```python
from build123d import *

# Parameters (mm, degrees)
SKETCH2_R                       = 10
BOSS_EXTRUDE1_DEPTH             = 12.7
TAP_DRILL_FOR_M3X0_5_TAP1_D     = 2.5
TAP_DRILL_FOR_M3X0_5_TAP1_DEPTH = 25
TAP_DRILL_FOR_M3X0_5_TAP1_TIP   = 0.751075774
M4X0_7_TAPPED_HOLE1_D           = 3.3
M4X0_7_TAPPED_HOLE1_DEPTH       = 14
M4X0_7_TAPPED_HOLE1_TIP         = 0.991420021


with BuildPart() as part:
    # Sketch2 → Boss-Extrude1 (new body)
    with BuildSketch(Plane.XY):
        with BuildLine():
            Line((27.5, 0), (-27.5, 0))
            Line((-27.5, 0), (-27.5, 22.5))
            ThreePointArc((-27.5, 22.5), (-24.571067812, 29.571067812), (-17.5, 32.5))
            Line((-17.5, 32.5), (17.5, 32.5))
            ThreePointArc((17.5, 32.5), (24.571067812, 29.571067812), (27.5, 22.5))
            Line((27.5, 22.5), (27.5, 0))
        make_face()
        with Locations((0, 14.5)):
            Circle(SKETCH2_R, mode=Mode.SUBTRACT)
    extrude(amount=BOSS_EXTRUDE1_DEPTH)

    # Tap Drill for M3x0.5 Tap1
    with Locations(Plane(origin=(13.522961568, 10.876533369, 0), x_dir=(-1, 0, 0), z_dir=(0, 0, -1))):
        with Locations((0, 0), (3.623466631, 13.522961568), (17.146428199, 17.146428199)):
            Hole(TAP_DRILL_FOR_M3X0_5_TAP1_D / 2, depth=TAP_DRILL_FOR_M3X0_5_TAP1_DEPTH)
            with Locations((0, 0, -(TAP_DRILL_FOR_M3X0_5_TAP1_DEPTH + TAP_DRILL_FOR_M3X0_5_TAP1_TIP / 2))):  # 118° drill point
                Cone(0, TAP_DRILL_FOR_M3X0_5_TAP1_D / 2, TAP_DRILL_FOR_M3X0_5_TAP1_TIP, mode=Mode.SUBTRACT)

    # M4x0.7 Tapped Hole1
    with Locations(Plane(origin=(22.25, 0, 6.35), x_dir=(0, 0, -1), z_dir=(0, -1, 0))):
        with Locations((0, 0), (0, -44.5)):
            Hole(M4X0_7_TAPPED_HOLE1_D / 2, depth=M4X0_7_TAPPED_HOLE1_DEPTH)
            with Locations((0, 0, -(M4X0_7_TAPPED_HOLE1_DEPTH + M4X0_7_TAPPED_HOLE1_TIP / 2))):  # 118° drill point
                Cone(0, M4X0_7_TAPPED_HOLE1_D / 2, M4X0_7_TAPPED_HOLE1_TIP, mode=Mode.SUBTRACT)


solid = part.part
```
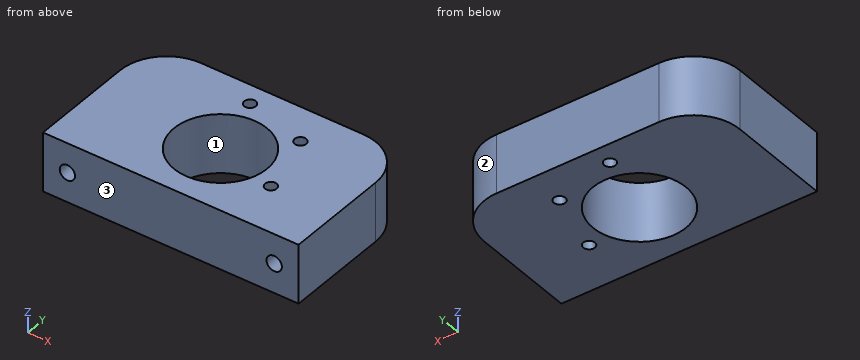
The listing builds one solid part. Answer for the finished solid, in the listing's coordinates (mm). Face numbers are marked on the shaded views. Coordinates: 2 decimals unless noted, no trailing zeros. Write each loop counter-clockwise with the first axis right and the second up, starting at its lowest first coordinate (ties: lowest second). Pieces come first, ordered by that corner, then holes.
Q1. The mould has two halves that part along X. Classify the marked faces 1, 2 and 3: released by +X, released by -X, zero draft, split by the parting line, or undercut.
Returned:
face 1: undercut
face 2: released by +X
face 3: zero draft
Q2. Section D-D, the plane z = 1 is taken. Write down the section's boundary in (x, y).
Returned:
outline: (-27.5, 0) - (27.5, 0) - (27.5, 22.5) arc R10 ccw to (17.5, 32.5) - (-17.5, 32.5) arc R10 ccw to (-27.5, 22.5) - close; hole circle Ø20 at (0, 14.5); hole circle Ø2.5 at (-3.62, 28.02); hole circle Ø2.5 at (9.9, 24.4); hole circle Ø2.5 at (13.52, 10.88)
Q3. Find the intervals of material crossed by line 1 along Z through (x, y) = (22.25, 7.25); line 2 along X through (y, z) = (11, 5); line 3 along X through (y, z) = (14, 12.25), in increasing order.
Returned:
line 1: z = 0 to 4.7, 8 to 12.7
line 2: x = -27.5 to -23.2, -21.3 to -9.37, 9.37 to 12.28, 14.77 to 21.3, 23.2 to 27.5
line 3: x = -27.5 to -9.99, 9.99 to 27.5
Q4. Section A-A, the plane x = 0 is taken. Write down the section's boundary in (y, z), then the cut area to 3 significant figures.
Returned:
outline: (0, 0) - (4.5, 0) - (4.5, 12.7) - (0, 12.7) - close; (24.5, 0) - (32.5, 0) - (32.5, 12.7) - (24.5, 12.7) - close
area: 159 mm2
Q5. Given P1, Ø3, axis at x = 13.52, y = 10.88, coming from the -Z side; P2, Ø4, axis at x = -22.25, z = 6.35, coming from the +Y side; P3, Ø18, axis at x = 0, y = 14.5, coming from the +Z side; P4, Ø4.5, axis at x = 22.25, z = 6.35, coming from the +Y side, each flat-ended and moving along its own axis, determine where each tip first touches the part or whether it passes through.
Returned:
P1: stops at z = 0
P2: stops at y = 32.11
P3: passes through
P4: stops at y = 32.18
Q6. Section B-B, the plane y = 7 is taken. Write down the section's boundary in (x, z), then the cut area to 3 significant figures.
Returned:
outline: (-27.5, 0) - (-6.61, 0) - (-6.61, 12.7) - (-27.5, 12.7) - close; (6.61, 0) - (27.5, 0) - (27.5, 12.7) - (6.61, 12.7) - close; hole circle Ø3.3 at (-22.25, 6.35); hole circle Ø3.3 at (22.25, 6.35)
area: 513 mm2
Q7. Section C-C, the plane y = 19 is taken. Write down the section's boundary in (x, z).
Returned:
outline: (-27.5, 0) - (-8.93, 0) - (-8.93, 12.7) - (-27.5, 12.7) - close; (8.93, 0) - (27.5, 0) - (27.5, 12.7) - (8.93, 12.7) - close
